Check sheet for the drawn part. Datum: minimum x, y, z corner. Units: mm. Give positions to 0.01 mm unless a question says otherwise; leave off trailing zeros. Write each loop counter-clockwise with the first axis right and the second up, starting at its lowest first coordinate (ties: lowest second). Pieces come first, ordered by that corner, then holes. Notation, with made-up numbers: M 44,-4.5 L 69,-4.5 A29 ccw 69,32.5 Z; hole C 51,30.5 d11. An arc over 180 degrees is marked long. Write item = value, one per line.
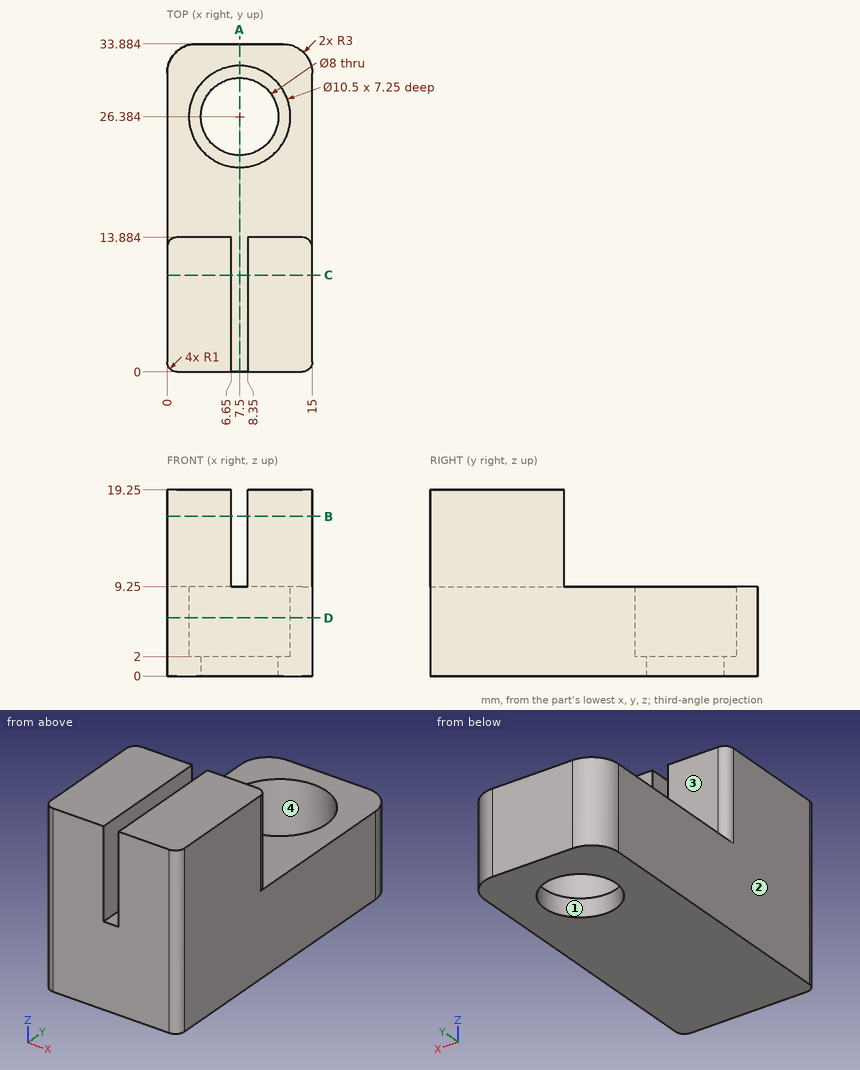
1) Draft check along X on the marked faces 1, 2, 3 and 4. Enter one of: +X half, -X half, draft (parallel to the pull), parting line (faces both ways), or undercut.
From the geometry:
face_1 = undercut
face_2 = -X half
face_3 = draft
face_4 = undercut
2) Cross-section at B-B on z = 16.5. Record the boundary of the cut face in (x, y).
From the geometry:
outline = M 0,1 A1 ccw 1,0 L 6.65,0 L 6.65,13.88 L 1,13.88 A1 ccw 0,12.88 Z; M 8.35,0 L 14,0 A1 ccw 15,1 L 15,12.88 A1 ccw 14,13.88 L 8.35,13.88 Z
3) Depth check by flat-ended pin: P1, Ø8.5, axis at x = 6.5, y = 27.5, coming from the +Z side; P2, Ø4.5, axis at x = 11, z = 12, coming from the +Y side; P3, Ø8.5, axis at x = 7.5, y = 26.38, coming from the +Z side. Enter the tip coordinate at first touch or a pass-through.
From the geometry:
P1 = 9.25
P2 = 13.88
P3 = 2
4) Cross-section at A-A on x = 7.5. Record the boundary of the cut face in (y, z), plus the area to 3 significant figures.
From the geometry:
outline = M 0,0 L 22.38,0 L 22.38,2 L 21.13,2 L 21.13,9.25 L 0,9.25 Z; M 30.38,0 L 33.88,0 L 33.88,9.25 L 31.63,9.25 L 31.63,2 L 30.38,2 Z
area = 221 mm^2
5) Material ranges on probe 1 along X at (y, z) = (2, 12.75); probe 2 along Y at (x, z) = (7.5, 1.5); probe 3 along Y at (x, z) = (7.5, 6.5), recorded low to high. Write a range as from..to.
From the geometry:
probe_1 = 0..6.65, 8.35..15
probe_2 = 0..22.38, 30.38..33.88
probe_3 = 0..21.13, 31.63..33.88
6) Cross-section at D-D on z = 6. Record the boundary of the cut face in (x, y).
From the geometry:
outline = M 0,1 A1 ccw 1,0 L 14,0 A1 ccw 15,1 L 15,30.88 A3 ccw 12,33.88 L 3,33.88 A3 ccw 0,30.88 Z; hole C 7.5,26.38 d10.5
7) Cross-section at C-C on y = 10. Record the boundary of the cut face in (x, z), plus the area to 3 significant figures.
From the geometry:
outline = M 0,0 L 15,0 L 15,19.25 L 8.35,19.25 L 8.35,9.25 L 6.65,9.25 L 6.65,19.25 L 0,19.25 Z
area = 272 mm^2
